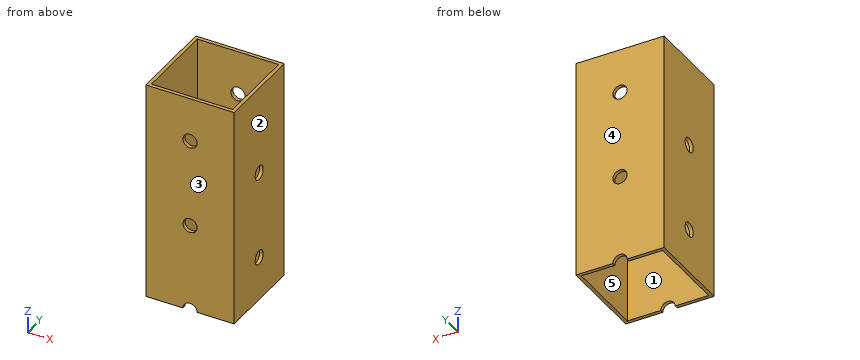
Autodesk Inventor part; units mm, degrees
ref_plane "YZ Plane" through (0, 0, 0) normal (1, 0, 0) x (0, 1, 0)
ref_plane "XZ Plane" through (0, 0, 0) normal (0, 1, 0) x (-1, 0, 0)
ref_plane "XY Plane" through (0, 0, 0) normal (0, 0, 1) x (1, 0, 0)
sketch "Sketch1" plane through (0, 0, 0) normal (0, 0, 1) x (1, 0, 0)
  line L0 (-12.7, -12.7) -> (12.7, -12.7)
  line L1 (12.7, -12.7) -> (12.7, 12.7)
  line L2 (12.7, 12.7) -> (-12.7, 12.7)
  line L3 (-12.7, 12.7) -> (-12.7, -12.7)
  line L4 (-12.7, -12.7) -> (12.7, 12.7) construction
  line L5 (12.7, -12.7) -> (-12.7, 12.7) construction
  line L6 (-11.684, 11.684) -> (11.684, 11.684)
  line L7 (11.684, 11.684) -> (11.684, -11.684)
  line L8 (11.684, -11.684) -> (-11.684, -11.684)
  line L9 (-11.684, -11.684) -> (-11.684, 11.684)
  point P0 (0, 0)
  dimension "l1" = 25.4
  dimension "l2" = 25.4
  dimension "wt" = 1.016
extrude "Extrusion1" add sketch "Sketch1" against normal blind 63.5
sketch "Sketch2" plane through (-12.7, 12.7, 0) normal (0, 1, 0) x (1, 0, 0)
  line L0 (25.4, 0) -> (0, 0)
  line L1 (25.4, 0) -> (25.4, 63.5)
  line L2 (0, 63.5) -> (25.4, 63.5)
  line L3 (0, 0) -> (0, 63.5)
  point P0 (12.7, 0)
  point P1 (12.7, 12.7)
  dimension "d5" = 25.4
  dimension "d6" = 12.7
  dimension "d7" = 12.7
hole "Hole3" at (0, 12.7, -12.7) direction (0, -1, 0) diameter 4.0894 end through all
sketch "Sketch3" plane through (12.7, -12.7, 0) normal (1, 0, 0) x (0, 0, -1)
  line L0 (0, 0) -> (0, 25.4)
  line L1 (0, 0) -> (63.5, 0)
  line L2 (63.5, 25.4) -> (63.5, 0)
  line L3 (0, 25.4) -> (63.5, 25.4)
  point P0 (0, 12.7)
  point P1 (25.4, 12.7)
  dimension "d22" = 25.4
  dimension "d23" = 12.7
  dimension "d24" = 25.4
hole "Hole4" at (12.7, 0, -25.4) direction (-1, 0, 0) diameter 4.0894 end through all
pattern_linear "Rectangular Pattern1" count 4 spacing 25.4 along (0, 0, -1) of "Hole3"
pattern_linear "Rectangular Pattern2" count 4 spacing 25.4 along (0, 0, -1) of "Hole4"
properties part number "versatubing_1x1x40" material "Aluminum 6061"
Verification items for the finished model (mm, model axes). Face numbers are marked on the shaded views. A direction names the side the tool comes from. Coordinates: 2 decimals unless noted, no trailing zeros. Order: outer loops, then holes, each group sorted by start corner. A loop starts at its lowest first (then second) coordinate and runs counter-clockwise, first axis right, second up.
1. Go/stop test with a flat-tipped pin: pin 1 Ø2 at (x, y) = (4.5, -10) entering from -Z. Record where the tip stops, or that it passes through.
Results found:
pin 1: passes through
2. Release check for a two-part mould opening along X. For the marked faces 1, 2 and 3 record: +X half, -X half, draft (parallel to the pull), parting line (faces both ways), or undercut.
Results found:
face 1: undercut
face 2: +X half
face 3: draft
3. Sectioned sample at C-C, the plane x = 0. Record the cut outline in (y, z).
Results found:
outline: (-12.7, -61.46) - (-11.68, -61.46) - (-11.68, -40.14) - (-12.7, -40.14) - close; (-12.7, -36.06) - (-11.68, -36.06) - (-11.68, -14.74) - (-12.7, -14.74) - close; (-12.7, -10.66) - (-11.68, -10.66) - (-11.68, 0) - (-12.7, 0) - close; (11.68, -61.46) - (12.7, -61.46) - (12.7, -40.14) - (11.68, -40.14) - close; (11.68, -36.06) - (12.7, -36.06) - (12.7, -14.74) - (11.68, -14.74) - close; (11.68, -10.66) - (12.7, -10.66) - (12.7, 0) - (11.68, 0) - close
4. Scan lines: line 1 (Z direction, x = 11.95, y = 0); line 2 (X direction, y = -0.25, z = -17.5); line 3 (Z direction, x = 0, y = 12.5). Record each from-to range of solid material in increasing order.
Results found:
line 1: z = -63.5 to -52.84, -48.76 to -27.44, -23.36 to 0
line 2: x = -12.7 to -11.68, 11.68 to 12.7
line 3: z = -61.46 to -40.14, -36.06 to -14.74, -10.66 to 0
5. Sectioned sample at D-D, the plane z = -5. Record the cut outline in (x, y), and give its area (3 significant figures).
Results found:
outline: (-12.7, -12.7) - (12.7, -12.7) - (12.7, 12.7) - (-12.7, 12.7) - close; hole (-11.68, -11.68) - (11.68, -11.68) - (11.68, 11.68) - (-11.68, 11.68) - close
area: 99.1 mm2
6. Sectioned sample at A-A, the plane z = -12.7. Record the cut outline in (x, y), and give its area (3 significant figures).
Results found:
outline: (-12.7, -12.7) - (-2.04, -12.7) - (-2.04, -11.68) - (-11.68, -11.68) - (-11.68, 11.68) - (-2.04, 11.68) - (-2.04, 12.7) - (-12.7, 12.7) - close; (2.04, -12.7) - (12.7, -12.7) - (12.7, 12.7) - (2.04, 12.7) - (2.04, 11.68) - (11.68, 11.68) - (11.68, -11.68) - (2.04, -11.68) - close
area: 90.8 mm2
7. Sectioned sample at B-B, the plane y = -4.75. Record the cut outline in (x, z).
Results found:
outline: (-12.7, -63.5) - (-11.68, -63.5) - (-11.68, 0) - (-12.7, 0) - close; (11.68, -63.5) - (12.7, -63.5) - (12.7, 0) - (11.68, 0) - close
8. Set-up check for the marked faces 4 and 5: record each of +Z, -Z, +X, -X, +Y, -Y from which the full face is reachable in a straight line by a thin tool's end or side.
Results found:
face 4: +Z, -Z, +X, -X, +Y
face 5: +Z, -Z
